Autodesk Inventor part; units mm, degrees
ref_plane "YZ Plane" through (0, 0, 0) normal (1, 0, 0) x (0, 1, 0)
ref_plane "XZ Plane" through (0, 0, 0) normal (0, 1, 0) x (-1, 0, 0)
ref_plane "XY Plane" through (0, 0, 0) normal (0, 0, 1) x (1, 0, 0)
sketch "Sketch1" plane through (0, 0, 0) normal (0, 0, 1) x (1, 0, 0)
  line L0 (3.8073, 0) -> (25.4, 0)
  line L1 (25.4, 0) -> (25.4, 25.4)
  line L2 (25.4, 25.4) -> (0, 25.4)
  line L3 (0, 25.4) -> (0, 3.8073)
  line L4 (0, 3.8073) -> (3.8073, 0)
  line L5 (0, 3.8073) -> (5.3843, 3.8073) construction
  point P0 (0, 0)
  dimension "d2" = 25.4
  dimension "d3" = 25.4
  dimension "d4" = 45
extrude "Extrusion1" add sketch "Sketch1" along normal blind 12.7
sketch "Sketch2" plane through (0, 25.4, 0) normal (0, 1, 0) x (1, 0, 0)
  line L0 (25.4, 0) -> (0, 0)
  line L1 (0, 0) -> (0, -12.7)
  line L2 (25.4, -12.7) -> (0, -12.7)
  line L3 (25.4, 0) -> (25.4, -12.7)
  line L4 (3.8073, 0) -> (3.8073, -12.7)
  circle A0 centre (3.8073, -6.35) radius 1.905
  dimension "d7" = 3.81
extrude "Extrusion2" add sketch "Sketch2" along normal blind 3.81 contours A0 L4 | L4 A0
properties part number "Finger Servo"
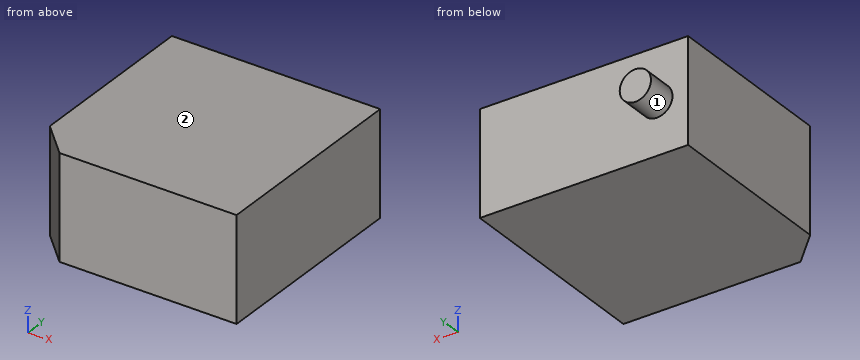
The model under review builds one solid part; all positions refer to its coordinate system, in mm. Face numbers are marked on the shaded views. A direction names the side the tool comes from. Give positions to 0.01 mm unless a question says otherwise; leave off trailing zeros. Loops run counter-clockwise (first coordinate to the right, second up) from the corner with the lowest first, then second, coordinate; pieces in that order, holes last. Notation, with made-up numbers: (79, 42) -> (95, 42) arc R26 ccw to (95, 66) -> close; hole circle Ø7 at (-27, -29). An arc over 180 degrees is marked (long way). Use CSV: the item, a comma, the result in double quotes.
1. Consider section B-B, the plane x = 5. Write out the cut boundary in (y, z), then the cut area to 3 significant figures.
Result:
outline,"(0, 0) -> (25.4, 0) -> (25.4, 4.86) -> (29.21, 4.86) -> (29.21, 7.84) -> (25.4, 7.84) -> (25.4, 12.7) -> (0, 12.7) -> close"
area,"334 mm²"
2. To check wall thickness, follow probe 1 along Y at (x, z) = (18.75, 7.5); probe 2 along X at (y, z) = (1.5, 8.75); probe 3 along Y at (x, z) = (2, 1.75). State the ranges of each line that lie inside material, in increasing order. Write a range as from..to.
Result:
probe 1,"y = 0..25.4"
probe 2,"x = 2.31..25.4"
probe 3,"y = 1.81..25.4"
3. For P1, Ø6, axis at x = 18.5, z = 10.5, coming from the +Y side, flat-tipped, find the tip position at first contact; note if it passes through.
Result:
P1,"stops at y = 25.4"
4. Consider section A-A, the plane z = 6.35. Write out the cut boundary in (x, y).
Result:
outline,"(0, 3.81) -> (3.81, 0) -> (25.4, 0) -> (25.4, 25.4) -> (5.71, 25.4) -> (5.71, 29.21) -> (1.9, 29.21) -> (1.9, 25.4) -> (0, 25.4) -> close"
5. Consider section D-D, the plane x = 21. Write out the cut boundary in (y, z).
Result:
outline,"(0, 0) -> (25.4, 0) -> (25.4, 12.7) -> (0, 12.7) -> close"
6. Consider section C-C, the plane z = 1.75. Write out the cut boundary in (x, y).
Result:
outline,"(0, 3.81) -> (3.81, 0) -> (25.4, 0) -> (25.4, 25.4) -> (0, 25.4) -> close"
7. Machinability: for the marked faces 1 and 2, which of the approach directions +Z, -Z, +X, -X, +Y, -Y give a long, thin tool a straight path to every point of the face, cutting with its end or side? Answer none if there is none.
Result:
face 1,"+Y"
face 2,"+Z, +X, -X, +Y, -Y"
